Here's how the part is built. I have some questions about the finished solid (model axes, mm). A direction names the side the tool comes from. Give positions to 0.01 mm unless a question says otherwise; leave off trailing zeros. Loops run counter-clockwise (first coordinate to the right, second up) from the corner with the lowest first, then second, coordinate; pieces in that order, holes last. Notation, with made-up numbers: (-11, 36.25) -> (-3, 36.25) arc R7 cw to (-3, 48.25) -> close; hole circle Ø7 at (41.25, 4). An arc over 180 degrees is marked (long way). Answer in a Markdown table with one row per item. Add a question column.
Item 1: Which directions (+Z, -Z, +X, -X, +Y, -Y) give clear straight access to the entire face, cutting with the end or side of a thin tool? Please do faces 1 (the face through (0, -2.15, -1)), 2 (the face through (4.81, 0, -1)), 3 (the face through (-3.41, 0.15, 4.42)), 4 (the face through (-0.1, -2.4, 0)), 5 (the face through (-4.81, 0, -1)).
Item 2: If we section it at C-C (z = 0.25): Give the number of separate pieces and of enclosed holes in the cut face, then the cut area to 3 significant figures.
Item 3: For P1, Ø3, axis at x = 7.15, y = 0, coming from the +Z side; P2, Ø1, axis at y = 0, z = 4, coming from the +X side; P3, Ø0.8, axis at y = 1, z = -1, coming from the -X side, each with a flat end and sliding along its axis, tell me the tip position at first contact or that it passes through.
Item 4: If I drill on line 1 (X direction, y = -0.55, z = -0.05); line 2 (Y direction, x = -1.25, z = 3); line 3 (Y direction, x = 7.15, z = 0.9), over which ranges is the centre line in solid material (lowest first)?
Item 5: If we section it at B-B (z = 6): Write out the boundary of the cut face in (x, y), then the cut area to 3 significant figures.
Item 6: If we section it at A-A (x = -7.15): Write out the boundary of the cut face in (y, z).
Item 7: We'd pull the mould along X, two halves only. Please class faces 6 (the face through (0, 2.7, 3)), 7 (the face through (0, 0, 2.5)), 8 (the face through (9.9, 0, 1)): released by +X, released by -X, zero draft, split by the parting line, or undercut.
```python
from build123d import *

# Parameters (mm, degrees)
SKETCH_1_W          = 19.8
SKETCH_1_H          = 5.4
SKETCH_1_R          = 1.15
EXTRUDE_1_DEPTH     = 2.5
FILLET_1_R          = 0.5
FILLET_2_R          = 0.5
SKETCH_3_W          = 9.62
SKETCH_3_H          = 4.3
EXTRUDE_2_DEPTH     = 2.6
SKETCH_4_R          = 0.31
CUT_EXTRUDE_1_DEPTH = 4.5
EXTRUDE_3_DEPTH     = 4.4
FILLET_3_R          = 0.5


with BuildPart() as part:
    # 草图1 → 凸台-拉伸1 (new body)
    with BuildSketch(Plane.XY):
        Rectangle(SKETCH_1_W, SKETCH_1_H)
        with Locations((-7.15, 0)):
            Circle(SKETCH_1_R, mode=Mode.SUBTRACT)
        with Locations(Location((7.15, 0, 0), (0, 0, 180))):
            Circle(SKETCH_1_R, mode=Mode.SUBTRACT)
    extrude(amount=EXTRUDE_1_DEPTH)

    # 圆角1
    fillet_1_edges = [part.edges().sort_by_distance(p)[0] for p in [
        (-9.9, 2.7, 1.25),
    ]]
    fillet(fillet_1_edges, radius=FILLET_1_R)

    # 圆角2
    fillet_2_edges = [part.edges().sort_by_distance(p)[0] for p in [
        (9.9, 2.7, 1.25),
        (9.9, -2.7, 1.25),
        (-9.9, -2.7, 1.25),
    ]]
    fillet(fillet_2_edges, radius=FILLET_2_R)

    # 草图3 → 凸台-拉伸2 (add)
    with BuildSketch(Plane(origin=(0, 0, 0), x_dir=(-1, 0, 0), z_dir=(0, 0, -1))):
        Rectangle(SKETCH_3_W, SKETCH_3_H)
    extrude(amount=EXTRUDE_2_DEPTH)

    # 草图4 → 切除-拉伸1 (cut)
    with BuildSketch(Plane(origin=(0, 0, -2.6), x_dir=(-1, 0, 0), z_dir=(0, 0, -1))):
        with Locations((-1.905, 0.55)):
            Circle(SKETCH_4_R)
        with Locations((-0.635, 0.55)):
            Circle(SKETCH_4_R)
        with Locations((0.635, 0.55)):
            Circle(SKETCH_4_R)
        with Locations((1.905, 0.55)):
            Circle(SKETCH_4_R)
        with Locations(Location((-2.54, -0.55, 0), (0, 0, 180))):
            Circle(SKETCH_4_R)
        with Locations(Location((-1.27, -0.55, 0), (0, 0, 180))):
            Circle(SKETCH_4_R)
        with Locations(Location((0, -0.55, 0), (0, 0, 180))):
            Circle(SKETCH_4_R)
        with Locations(Location((1.27, -0.55, 0), (0, 0, 180))):
            Circle(SKETCH_4_R)
        with Locations(Location((2.54, -0.55, 0), (0, 0, 180))):
            Circle(SKETCH_4_R)
    extrude(amount=-CUT_EXTRUDE_1_DEPTH, mode=Mode.SUBTRACT)

    # 草图5 → 凸台-拉伸3 (add)
    with BuildSketch(Plane.XY.offset(2.5)):
        with BuildLine():
            Line((-2.651993332, 2.7), (2.651993332, 2.7))
            ThreePointArc((2.651993332, 2.7), (2.937625447, 2.610383107), (3.120867712, 2.373657178))
            Line((3.120867712, 2.373657178), (4.750497342, -2.026342822))
            ThreePointArc((4.750497342, -2.026342822), (4.692006068, -2.485632116), (4.281622961, -2.7))
            Line((4.281622961, -2.7), (-4.281622961, -2.7))
            ThreePointArc((-4.281622961, -2.7), (-4.692006068, -2.485632116), (-4.750497342, -2.026342822))
            Line((-4.750497342, -2.026342822), (-3.120867712, 2.373657178))
            ThreePointArc((-3.120867712, 2.373657178), (-2.937625447, 2.610383107), (-2.651993332, 2.7))
        make_face()
        with BuildLine():
            Line((-2.303986663, 2.2), (2.303986663, 2.2))
            ThreePointArc((2.303986663, 2.2), (2.589618779, 2.110383107), (2.772861043, 1.873657178))
            Line((2.772861043, 1.873657178), (4.032120303, -1.526342822))
            ThreePointArc((4.032120303, -1.526342822), (3.973629029, -1.985632116), (3.563245922, -2.2))
            Line((3.563245922, -2.2), (-3.563245922, -2.2))
            ThreePointArc((-3.563245922, -2.2), (-3.973629029, -1.985632116), (-4.032120303, -1.526342822))
            Line((-4.032120303, -1.526342822), (-2.772861043, 1.873657178))
            ThreePointArc((-2.772861043, 1.873657178), (-2.589618779, 2.110383107), (-2.303986663, 2.2))
        make_face(mode=Mode.SUBTRACT)
    extrude(amount=EXTRUDE_3_DEPTH)

    # 圆角3
    fillet_3_edges = [part.edges().sort_by_distance(p)[0] for p in [
        (-3.973629029, -1.985632116, 6.9),
        (0, -2.2, 6.9),
        (3.973629029, -1.985632116, 6.9),
        (3.402490673, 0.173657178, 6.9),
        (2.589618779, 2.110383107, 6.9),
        (0, 2.2, 6.9),
        (-2.589618779, 2.110383107, 6.9),
        (-3.402490673, 0.173657178, 6.9),
    ]]
    fillet(fillet_3_edges, radius=FILLET_3_R - 0.0001)  # a hair under: the kernel refuses the full size


solid = part.part
```
Recorded:
| question | item | result |
|---|---|---|
| 1 | face 1 | -Z, +X, -X, -Y |
| 1 | face 2 | -Z, +X, +Y, -Y |
| 1 | face 3 | +Z |
| 1 | face 4 | -Z |
| 1 | face 5 | -Z, -X, +Y, -Y |
| 2 | separate pieces | 1 |
| 2 | enclosed holes | 11 |
| 2 | area | 95.7 mm^2 |
| 3 | P1 | stops at z = 2.5 |
| 3 | P2 | stops at x = 4.19 |
| 3 | P3 | stops at x = -4.81 |
| 4 | line 1 | x = -4.81 to -2.85, -2.23 to -1.58, -0.96 to -0.31, 0.31 to 0.96, 1.58 to 2.23, 2.85 to 4.81 |
| 4 | line 2 | y = -2.7 to -2.2, 2.2 to 2.7 |
| 4 | line 3 | y = -2.7 to -1.15, 1.15 to 2.7 |
| 5 | outline | (-4.75, -2.03) arc R0.5 ccw to (-4.28, -2.7) -> (4.28, -2.7) arc R0.5 ccw to (4.75, -2.03) -> (3.12, 2.37) arc R0.5 ccw to (2.65, 2.7) -> (-2.65, 2.7) arc R0.5 ccw to (-3.12, 2.37) -> close; hole (-4.03, -1.53) arc R0.5 ccw to (-3.56, -2.2) -> (3.56, -2.2) arc R0.5 ccw to (4.03, -1.53) -> (2.77, 1.87) arc R0.5 ccw to (2.3, 2.2) -> (-2.3, 2.2) arc R0.5 ccw to (-2.77, 1.87) -> close |
| 5 | area | 12.7 mm^2 |
| 6 | outline | (-2.7, 0) -> (-1.15, 0) -> (-1.15, 2.5) -> (-2.7, 2.5) -> close; (1.15, 0) -> (2.7, 0) -> (2.7, 2.5) -> (1.15, 2.5) -> close |
| 7 | face 6 | zero draft |
| 7 | face 7 | undercut |
| 7 | face 8 | released by +X |
